Model file for the job. Use its own axes, mm. A direction names the side the tool comes from. Give positions to 0.01 mm unless a question says otherwise; leave off trailing zeros. Loops run counter-clockwise (first coordinate to the right, second up) from the corner with the lowest first, then second, coordinate; pieces in that order, holes last. Notation, with made-up numbers: M -16,80 L 42,80 A26 ccw 42,102 Z; hole C 56,-29.75 d10. An arc over 180 degrees is marked long. Answer in a Markdown table with one row per item.
```python
from build123d import *

# Parameters (mm, degrees)
BOSS_EXTRUDE1_DEPTH     = 50.8
SKETCH2_W               = 74.235303162
SKETCH2_H               = 25.4
CUT_EXTRUDE1_DEPTH      = 104.175287739
FILLET2_R               = 12.7
SKETCH4_R               = 6.477
CUT_EXTRUDE2_DEPTH      = 105.147743615
F_1_2_20_TAPPED_HOLE1_D = 11.50874


with BuildPart() as part:
    # Sketch1 → Boss-Extrude1 (new, symmetric)
    with BuildSketch(Plane.XY):
        Polygon((0, 0), (-37.117651581, 0), (-44.45, 12.7), (-88.9, 12.7), (-88.9, 6.35), (-48.116174209, 6.35), (-40.783825791, -6.35), (40.783825791, -6.35), (48.116174209, 6.35), (88.9, 6.35), (88.9, 12.7), (44.45, 12.7), (37.117651581, 0), align=None)
    extrude(amount=BOSS_EXTRUDE1_DEPTH, both=True)

    # Sketch2 → Cut-Extrude1 (cut, through all)
    with BuildSketch(Plane(origin=(0, 0, 0), x_dir=(1, 0, 0), z_dir=(0, 1, 0))):
        with Locations((0, 38.1)):
            Rectangle(SKETCH2_W, SKETCH2_H)
        Polygon((-37.117651581, -38.1), (-25.4, -38.1), (-12.7, -25.4), (12.7, -25.4), (25.4, -38.1), (37.117651581, -38.1), (37.117651581, -50.8), (-37.117651581, -50.8), align=None)
        with BuildLine():
            Line((-22.225, 6.35), (22.225, 6.35))
            ThreePointArc((22.225, 6.35), (28.575, 0), (22.225, -6.35))
            Line((22.225, -6.35), (-22.225, -6.35))
            ThreePointArc((-22.225, -6.35), (-28.575, 0), (-22.225, 6.35))
        make_face()
    extrude(amount=-CUT_EXTRUDE1_DEPTH, mode=Mode.SUBTRACT)

    # Fillet2
    fillet2_edges = [part.edges().sort_by_distance(p)[0] for p in [
        (88.9, 9.525, -50.8),
        (-88.9, 9.525, -50.8),
        (-88.9, 9.525, 50.8),
        (88.9, 9.525, 50.8),
    ]]
    fillet(fillet2_edges, radius=FILLET2_R)

    # Sketch4 → Cut-Extrude2 (cut, through all)
    with BuildSketch(Plane(origin=(0, 12.7, 0), x_dir=(1, 0, 0), z_dir=(0, 1, 0))):
        with Locations(Location((-57.15, 38.1, 0), (0, 0, 180))):
            Circle(SKETCH4_R)
        with Locations(Location((-57.15, -38.1, 0), (0, 0, 180))):
            Circle(SKETCH4_R)
        with Locations(Location((57.15, -38.1, 0), (0, 0, 180))):
            Circle(SKETCH4_R)
        with Locations(Location((57.15, 38.1, 0), (0, 0, 180))):
            Circle(SKETCH4_R)
    extrude(amount=-CUT_EXTRUDE2_DEPTH, mode=Mode.SUBTRACT)

    # 1/2-20 Tapped Hole1 (through all)
    with Locations(Plane(origin=(0, 12.7, 0), x_dir=(1, 0, 0), z_dir=(0, 1, 0))):
        with Locations((-76.2, 38.1), (-76.2, -38.1), (76.2, -38.1), (76.2, 38.1)):
            Hole(F_1_2_20_TAPPED_HOLE1_D / 2)


solid = part.part
```
Q1. Probe probe 1 along Z at (x, y) = (-57.15, 9.5); probe 2 along Z at (x, y) = (-76.2, 8.5); probe 3 along X at (y, z) = (11.5, -41). List the from-to ranges inside material, lowest first.
Reported:
| item | result |
|---|---|
| probe 1 | -50.8 to -44.58, -31.62 to 31.62, 44.58 to 50.8 |
| probe 2 | -50.8 to -43.85, -32.35 to 32.35, 43.85 to 50.8 |
| probe 3 | -88.56 to -81.17, -71.23 to -62.94, -51.36 to -43.76, 43.76 to 51.36, 62.94 to 71.23, 81.17 to 88.56 |
Q2. Saw through at A-A (z = 0). Give the cut face in (x, y) (3 decimals).
Reported:
| item | result |
|---|---|
| outline | M -88.9,6.35 L -48.116,6.35 L -40.784,-6.35 L -28.575,-6.35 L -28.575,0 L -37.118,0 L -44.45,12.7 L -88.9,12.7 Z; M 28.575,-6.35 L 40.784,-6.35 L 48.116,6.35 L 88.9,6.35 L 88.9,12.7 L 44.45,12.7 L 37.118,0 L 28.575,0 Z |
Q3. 3-axis set-ups, long thin cutter, end or side, ignore diameter. For faces 1 (the face through (-37.118, -3, 45)), 2 (the face through (0, -3, -6.35)), 3 (the face through (37.118, -3, -38)): which of +Z, -Z, +X, -X, +Y, -Y reach the whole face in a straight line?
Reported:
| item | result |
|---|---|
| face 1 | +Z, +Y, -Y |
| face 2 | +Y, -Y |
| face 3 | -Z, +Y, -Y |
Q4. Saw through at C-C (y = 9). Give the number of separate pieces and of enclosed holes in the cut face, and give its area (3 significant figures).
Reported:
| item | result |
|---|---|
| separate pieces | 2 |
| enclosed holes | 8 |
| area | 8,380 mm² |
Q5. Saw through at B-B (x = 57.15). Give the cut face in (y, z), and give its area (3 significant figures).
Reported:
| item | result |
|---|---|
| outline | M 6.35,-50.8 L 12.7,-50.8 L 12.7,-44.58 L 6.35,-44.58 Z; M 6.35,-31.62 L 12.7,-31.62 L 12.7,31.62 L 6.35,31.62 Z; M 6.35,44.58 L 12.7,44.58 L 12.7,50.8 L 6.35,50.8 Z |
| area | 481 mm² |
Q6. Mould opens along Z. For faces 4 (the face through (57.993, 9.569, 44.522)), 5 (the face through (44.4, -0.09, 0.71)), 6 (the face through (56, 8, 50.8)) say: released by +Z, released by -Z, zero draft, split by the parting line, or undercut.
Reported:
| item | result |
|---|---|
| face 4 | undercut |
| face 5 | zero draft |
| face 6 | released by +Z |
Q7. Saw through at D-D (x = -16). Give the cut face in (y, z).
Reported:
| item | result |
|---|---|
| outline | M -6.35,-25.4 L 0,-25.4 L 0,-6.35 L -6.35,-6.35 Z; M -6.35,6.35 L 0,6.35 L 0,28.7 L -6.35,28.7 Z |
Q8. Drop flat-ended pins along their axis: pin 1 (1.5 mm diameter, centred on y = -1.5, z = 16.5, fed in from +X); pin 2 (7 mm diameter, centred on x = 8.5, y = -3, fed in from +Z); pin 3 (13 mm diameter, centred on x = -76.2, z = 38.1, fed in from -Y). Give the stop position or say it passes through.
Reported:
| item | result |
|---|---|
| pin 1 | x = 44.02 |
| pin 2 | z = 25.4 |
| pin 3 | y = 6.35 |
